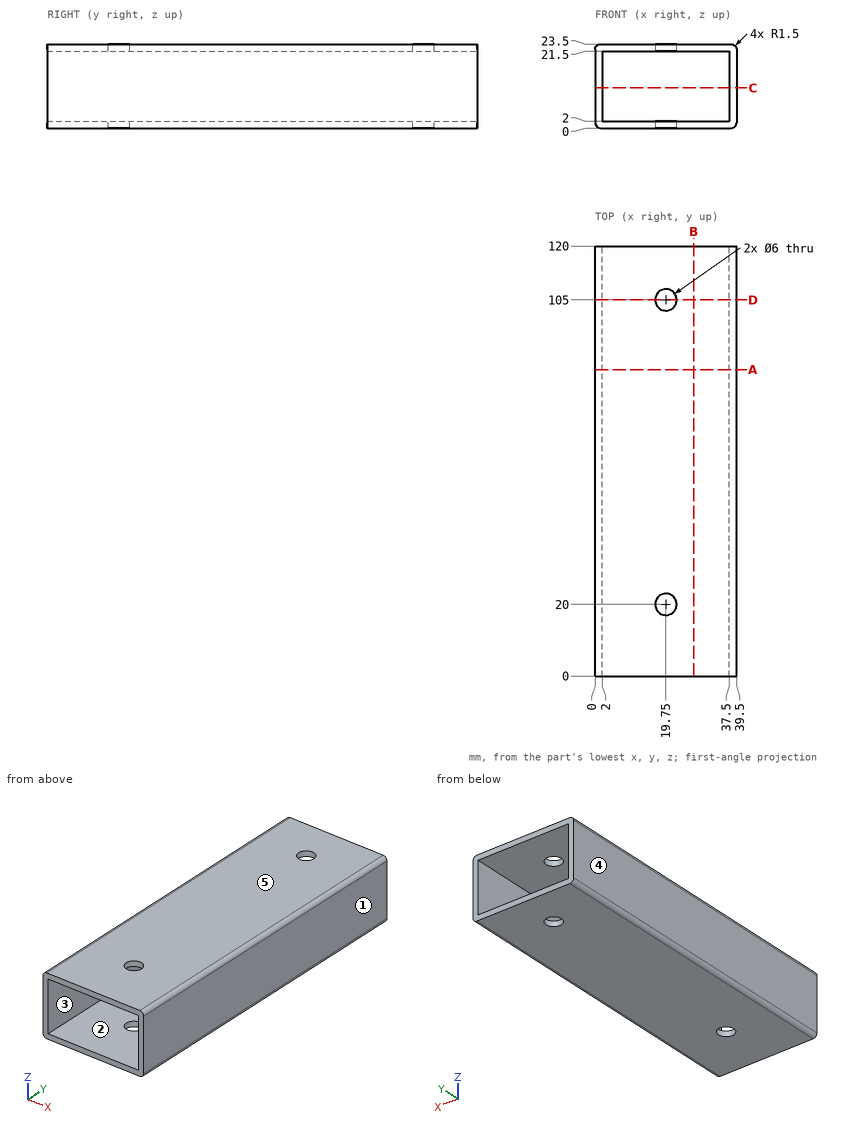
Print and shaded views of the part. All mm, measured from the part's lowest x, y and z. A direction names the side the tool comes from. Round coordinates to 2 decimals unless told otherwise and drop trailing zeros. Order: outer loops, then holes, each group sorted by start corner. A loop starts at its lowest first (then second) coordinate and runs counter-clockwise, first axis right, second up. Notation, with made-up numbers: (7, 12) - (46, 12) arc R18 cw to (46, 36) - close; hole circle Ø9 at (-19.75, 28). An arc over 180 degrees is marked (long way). Use a Markdown table: item, result.
1) Tool access for the marked faces 1 and 2: list every direction of +Z, -Z, +X, -X, +Y, -Y with a clear straight run to the whole face (end or side of a thin tool).
Recorded:
| item | result |
|---|---|
| face 1 | +Z, -Z, +X, +Y, -Y |
| face 2 | +Y, -Y |
2) Wall check: L1, parallel to Y at x = 19.75, z = 22.65; L2, parallel to X at y = 42.5, z = 19.5; L3, parallel to Z at x = 15.5, y = 108. Give the ranges that are in metal, low to high.
Recorded:
| item | result |
|---|---|
| L1 | y = 0 to 17, 23 to 102, 108 to 120 |
| L2 | x = 0 to 2, 37.5 to 39.5 |
| L3 | z = 0 to 2, 21.5 to 23.5 |
3) Pull direction X, two halves, no side cores. Call the marked faces 3, 4 and 5: pulls with the +X half, pulls with the -X half, needs draft (parallel to the pull), parting line crosses it, or undercut.
Recorded:
| item | result |
|---|---|
| face 3 | undercut |
| face 4 | pulls with the -X half |
| face 5 | needs draft |
4) Saw through at A-A on y = 85.5. Write the cut outline in (x, z), and give its area (3 significant figures).
Recorded:
| item | result |
|---|---|
| outline | (0, 1.5) arc R1.5 ccw to (1.5, 0) - (38, 0) arc R1.5 ccw to (39.5, 1.5) - (39.5, 22) arc R1.5 ccw to (38, 23.5) - (1.5, 23.5) arc R1.5 ccw to (0, 22) - close; hole (2, 2) - (37.5, 2) - (37.5, 21.5) - (2, 21.5) - close |
| area | 234 mm² |
5) Saw through at B-B on x = 27.5. Write the cut outline in (y, z).
Recorded:
| item | result |
|---|---|
| outline | (0, 0) - (120, 0) - (120, 2) - (0, 2) - close; (0, 21.5) - (120, 21.5) - (120, 23.5) - (0, 23.5) - close |
6) Saw through at C-C on z = 11.25. Write the cut outline in (x, y).
Recorded:
| item | result |
|---|---|
| outline | (0, 0) - (2, 0) - (2, 120) - (0, 120) - close; (37.5, 0) - (39.5, 0) - (39.5, 120) - (37.5, 120) - close |
7) Saw through at D-D on y = 105. Write the cut outline in (x, z).
Recorded:
| item | result |
|---|---|
| outline | (0, 1.5) arc R1.5 ccw to (1.5, 0) - (16.75, 0) - (16.75, 2) - (2, 2) - (2, 21.5) - (16.75, 21.5) - (16.75, 23.5) - (1.5, 23.5) arc R1.5 ccw to (0, 22) - close; (22.75, 0) - (38, 0) arc R1.5 ccw to (39.5, 1.5) - (39.5, 22) arc R1.5 ccw to (38, 23.5) - (22.75, 23.5) - (22.75, 21.5) - (37.5, 21.5) - (37.5, 2) - (22.75, 2) - close |
